The listing builds one solid part. Answer for the finished solid, in the listing's coordinates (mm). Round coordinates to 2 decimals unless told otherwise and drop trailing zeros. Order: outer loops, then holes, each group sorted by start corner. A loop starts at its lowest first (then second) coordinate and runs counter-clockwise, first axis right, second up. Notation, with made-up numbers: (12.5, 88) -> (17.5, 88) arc R21 ccw to (17.5, 96) -> close; hole circle Ø5 at (-39, 57.5). An arc over 180 degrees is marked (long way). Return JSON: item names as keys, results as strings. Group by question number.
(1) Consider line 1 (X direction, y = 44, z = 23.5); line 2 (X direction, y = 21, z = 43); line 3 (Y direction, x = 9, z = 39). Determine where each line is inside the solid, lowest interval first. Write a range as [from, to].
(2) The part is cut by section A-A (y = -1). Determine the outline of the cut face in (x, z), plus the area to 3 significant figures.
(3) Each of these flat-tipped pins is pushed along its axis until it touches: pin 1 (6 mm diameter, centred on y = 34, z = 39, fed in from +X); pin 2 (1 mm diameter, centred on x = -41.5, z = 32.5, fed in from +Y); pin 3 (2 mm diameter, centred on y = 44, z = 27.5, fed in from +X). Where does it stop, or does it pass through?
(4) The part is cut by section D-D (z = 43). Determine the outline of the cut face in (x, y), plus the area to 3 significant figures.
(5) The part is cut by section B-B (x = -56.5). Determine the outline of the cut face in (y, z).
(6) The part is cut by section C-C (z = 35). Determine the outline of the cut face in (x, y).
from build123d import *

# Parameters (mm, degrees)
F0_W     = 127
F0_H     = 35.337034
F1_DEPTH = 88.9
F2_R     = 25.4
F3_R     = 25.4
F4_R     = 25.4
F5_R     = 25.4


with BuildPart() as f1:
    # F0 (on Right) → F1 (new body, symmetric)
    with BuildSketch(Plane.YZ):
        with Locations((-5.457316, 29.881938)):
            Rectangle(F0_W, F0_H)
    extrude(amount=F1_DEPTH, both=True)

    # F2
    f2_edges = [f1.edges().sort_by_distance(p)[0] for p in [
        (-88.9, -5.457316, 47.550455),
    ]]
    fillet(f2_edges, radius=F2_R)

    # F3
    f3_edges = [f1.edges().sort_by_distance(p)[0] for p in [
        (88.9, -5.457316, 47.550455),
    ]]
    fillet(f3_edges, radius=F3_R)

    # F4
    f4_edges = [f1.edges().sort_by_distance(p)[0] for p in [
        (-88.9, 58.042684, 17.181938),
    ]]
    fillet(f4_edges, radius=F4_R)

    # F5
    f5_edges = [f1.edges().sort_by_distance(p)[0] for p in [
        (-88.9, -68.957316, 17.181938),
    ]]
    fillet(f5_edges, radius=F5_R)


solid = f1.part
Answer below:
{
 "1": {"line 1": "x = [-86.18, 86.18]", "line 2": "x = [-78.01, 78.01]", "line 3": "y = [-62.56, 51.65]"},
 "2": {"outline": "(-88.9, 12.21) -> (88.9, 12.21) -> (88.9, 22.15) arc R25.4 ccw to (63.5, 47.55) -> (-63.5, 47.55) arc R25.4 ccw to (-88.9, 22.15) -> close", "area": "6,010 mm²"},
 "3": {"pin 1": "stops at x = 84.76", "pin 2": "stops at y = 56.06", "pin 3": "stops at x = 86.12"},
 "4": {"outline": "(-78.01, -43.56) arc R14.51 ccw to (-63.5, -58.06) -> (63.5, -58.06) arc R14.51 ccw to (78.01, -43.56) -> (78.01, 32.64) arc R14.51 ccw to (63.5, 47.15) -> (-63.5, 47.15) arc R14.51 ccw to (-78.01, 32.64) -> close", "area": "16,200 mm²"},
 "5": {"outline": "(-68.96, 12.21) -> (58.04, 12.21) -> (58.04, 22.15) arc R25.4 ccw to (32.64, 47.55) -> (-43.56, 47.55) arc R25.4 ccw to (-68.96, 22.15) -> close"},
 "6": {"outline": "(-85.41, -43.56) arc R21.91 ccw to (-63.5, -65.47) -> (63.5, -65.47) arc R21.91 ccw to (85.41, -43.56) -> (85.41, 32.64) arc R21.91 ccw to (63.5, 54.55) -> (-63.5, 54.55) arc R21.91 ccw to (-85.41, 32.64) -> close"}
}
